Study the drawing (mm; zero at the part's minimum x, y, z) and answer. A direction names the side the tool comes from. Coordinates: 2 decimals unless noted, no trailing zeros. Write each loop counter-clockwise with the first axis right and the second up, starting at its lowest first coordinate (ties: lowest second). Pieces come first, ordered by that corner, then holes. Notation, with made-up numbers: (28.5, -33.5) - (74.5, -33.5) arc R26 cw to (74.5, -10.5) - close; hole circle Ø11 at (23.5, 24). An arc over 180 degrees is marked (long way). One line per item, written item: value.
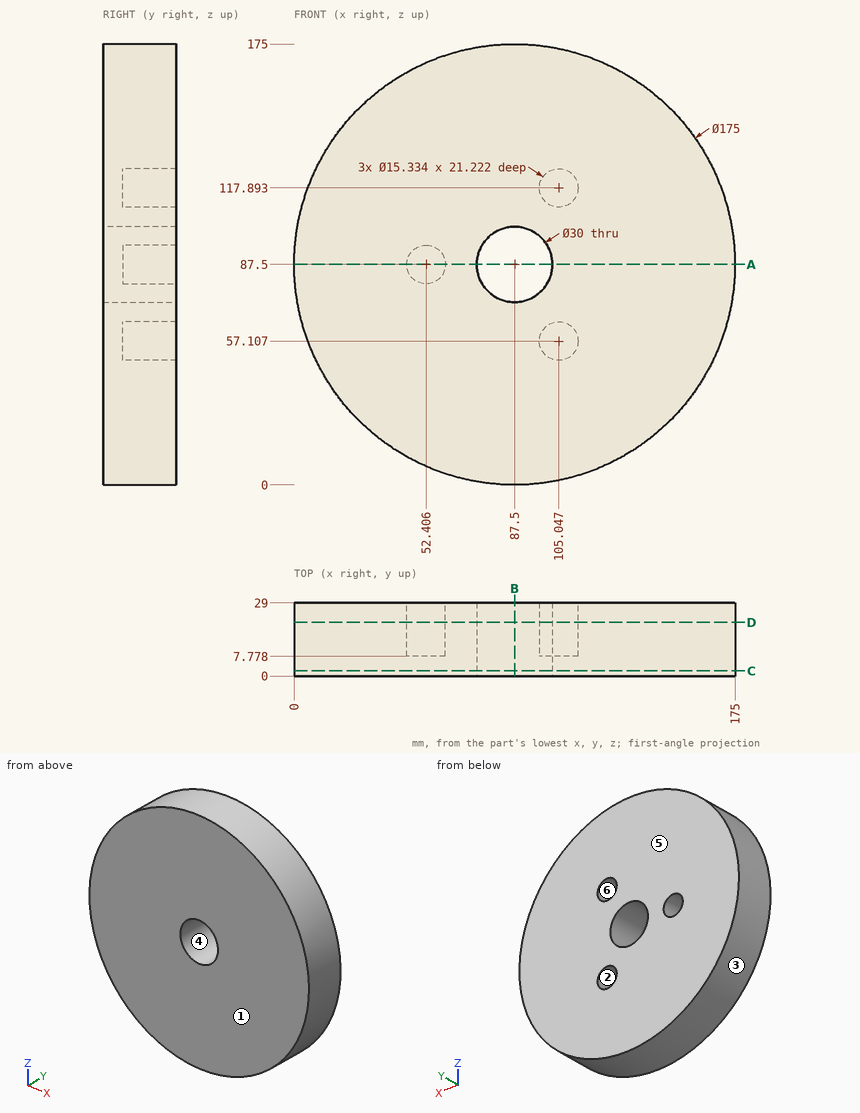
Item 1: Consider probe 1 along X at (y, z) = (17.25, 87.5); probe 2 along Z at (x, y) = (105.5, 23.5); probe 3 along Z at (x, y) = (77, 22.75). Determine where each line is inside the solid, lowest interval first.
Evaluation:
probe 1: x = 0 to 44.74, 60.07 to 72.5, 102.5 to 175
probe 2: z = 1.87 to 49.45, 64.76 to 110.24, 125.55 to 173.13
probe 3: z = 0.63 to 76.79, 98.21 to 174.37
Item 2: Section B-B, the plane x = 87.5 is taken. Determine the outline of the cut face in (y, z).
Evaluation:
outline: (0, 0) - (29, 0) - (29, 72.5) - (0, 72.5) - close; (0, 102.5) - (29, 102.5) - (29, 175) - (0, 175) - close
Item 3: Given pin 1 (8 mm diameter, centred on x = 156.5, y = 23.5, fed in from +Z); pin 2 (9 mm diameter, centred on x = 105.05, z = 57.11, fed in from -Y); pin 3 (2 mm diameter, centred on y = 4.5, z = 108.5, fed in from +X); pin 4 (6 mm diameter, centred on x = 95.5, y = 6.5, fed in from +Z), each flat-ended and moving along its own axis, determine where each tip first touches the part or whether it passes through.
Evaluation:
pin 1: stops at z = 146.08
pin 2: stops at y = 0
pin 3: stops at x = 172.68
pin 4: stops at z = 174.86
Item 4: Which of the six approach directions +Z, -Z, +X, -X, +Y, -Y give full straight-line access (tool end or side, diameter ignored) to the marked faces 1 and 2?
Evaluation:
face 1: +Z, -Z, +X, -X, -Y
face 2: +Y
Item 5: Section C-C, the plane y = 2 is taken. Determine the outline of the cut face in (x, z).
Evaluation:
outline: circle Ø175 at (87.5, 87.5); hole circle Ø30 at (87.5, 87.5)
Item 6: Determine the mould class of the marked faces 3, 4, 5 and 6 for opening direction Z: +Z half, -Z half, draft (parallel to the pull), parting line (faces both ways), or undercut.
Evaluation:
face 3: parting line
face 4: undercut
face 5: draft
face 6: undercut
Item 7: Section A-A, the plane z = 87.5 is taken. Determine the outline of the cut face in (x, y), then the cut area to 3 significant figures.
Evaluation:
outline: (0, 0) - (72.5, 0) - (72.5, 29) - (60.07, 29) - (60.07, 7.78) - (44.74, 7.78) - (44.74, 29) - (0, 29) - close; (102.5, 0) - (175, 0) - (175, 29) - (102.5, 29) - close
area: 3,880 mm2
Item 8: Section D-D, the plane y = 21.25 is taken. Determine the outline of the cut face in (x, z) (1 decimal), then the cut area to 3 significant figures.
Evaluation:
outline: circle Ø175 at (87.5, 87.5); hole circle Ø15.3 at (52.4, 87.5); hole circle Ø30 at (87.5, 87.5); hole circle Ø15.3 at (105, 57.1); hole circle Ø15.3 at (105, 117.9)
area: 22,800 mm2
